Job drawing, mm, ordinate dimensions from the low corner. One solid piece. A direction names the side the tool comes from. Coordinates: 2 decimals unless noted, no trailing zeros. Write each loop counter-clockwise with the first axis right and the second up, starting at its lowest first coordinate (ties: lowest second). Pieces come first, ordered by that corner, then holes.
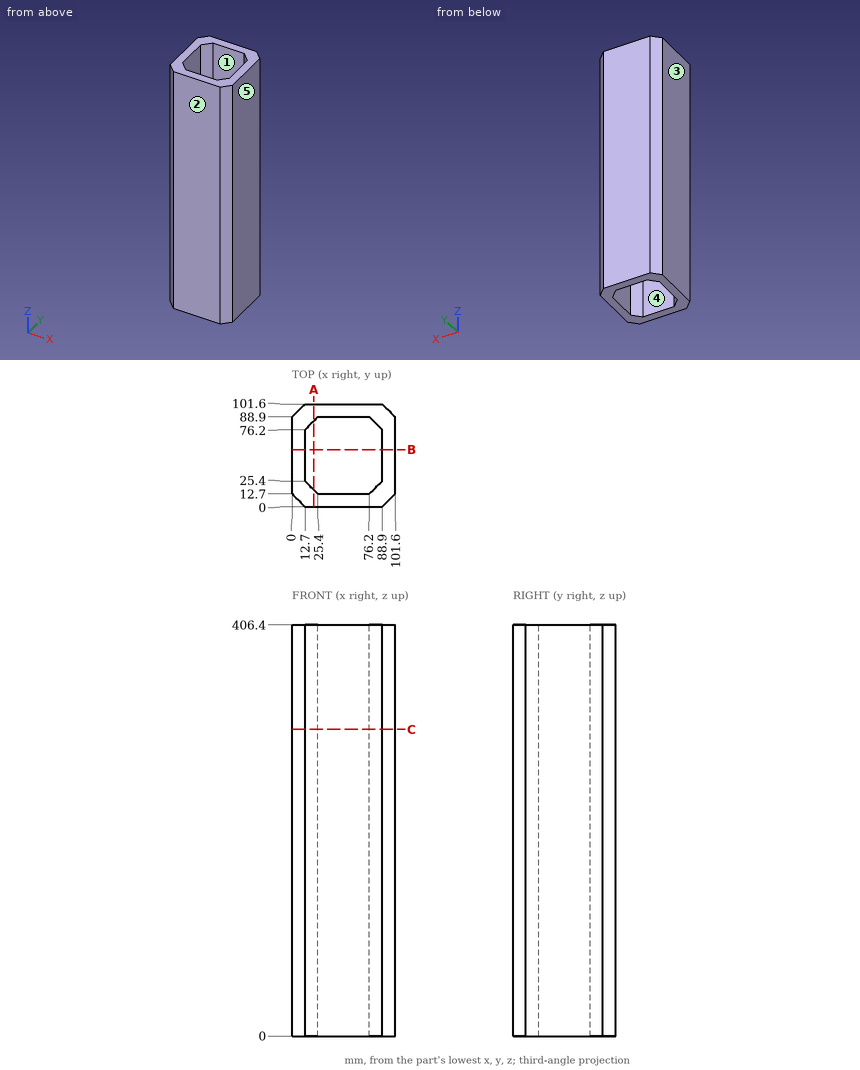
1. Saw through at A-A on x = 21.5. List the corners of the cut face in (y, z).
Computed values:
outline: (0, 0) - (16.6, 0) - (16.6, 406.4) - (0, 406.4) - close; (85, 0) - (101.6, 0) - (101.6, 406.4) - (85, 406.4) - close
2. Saw through at B-B on y = 56.5. List the corners of the cut face in (x, z), plus the area to 3 significant figures.
Computed values:
outline: (0, 0) - (12.7, 0) - (12.7, 406.4) - (0, 406.4) - close; (88.9, 0) - (101.6, 0) - (101.6, 406.4) - (88.9, 406.4) - close
area: 10,300 mm2
3. Mould opens along Y. For the marked faces 1, 2 and 3 say: +Y half, -Y half, draft (parallel to the pull), parting line (faces both ways), or undercut.
Computed values:
face 1: undercut
face 2: -Y half
face 3: draft
4. Saw through at C-C on z = 303. List the corners of the cut face in (x, y), plus the area to 3 significant figures.
Computed values:
outline: (0, 12.7) - (12.7, 0) - (88.9, 0) - (101.6, 12.7) - (101.6, 88.9) - (88.9, 101.6) - (12.7, 101.6) - (0, 88.9) - close; hole (12.7, 25.4) - (25.4, 12.7) - (76.2, 12.7) - (88.9, 25.4) - (88.9, 76.2) - (76.2, 88.9) - (25.4, 88.9) - (12.7, 76.2) - close
area: 4,520 mm2
5. Probe line 1 along Y through (x, z) = (71.5, 347); line 2 along X through (y, z) = (14.5, 333). List the from-to ranges inside material, lowest first.
Computed values:
line 1: y = 0 to 12.7, 88.9 to 101.6
line 2: x = 0 to 23.6, 78 to 101.6
6. 3-axis set-ups, long thin cutter, end or side, ignore diameter. For the marked faces 4 and 5: which of +Z, -Z, +X, -X, +Y, -Y reach the whole face in a straight line?
Computed values:
face 4: +Z, -Z
face 5: +Z, -Z, +X, +Y, -Y
7. Flat gauge pins, fed straight in: pin 1 (2 mm diameter, centred on x = 19, y = 85, fed in from -Z); pin 2 (1.5 mm diameter, centred on x = 10.5, z = 133, fed in from +Y). Where does each tip first touch, or does it go through?
Computed values:
pin 1: stops at z = 0
pin 2: stops at y = 100.15
